from build123d import *

# Parameters (mm, degrees)
SKETCH1_R           = 9
SKETCH1_R_2         = 4
BOSS_EXTRUDE1_DEPTH = 5
SKETCH2_W           = 5
SKETCH2_H           = 10
CUT_EXTRUDE3_DEPTH  = 3
CIRPATTERN1_COUNT   = 6
SKETCH3_R           = 4.05
BOSS_EXTRUDE2_DEPTH = 3


with BuildPart() as part:
    # Sketch1 → Boss-Extrude1 (new body, symmetric)
    with BuildSketch(Plane.XY):
        Circle(SKETCH1_R)
        Circle(SKETCH1_R_2, mode=Mode.SUBTRACT)
    extrude(amount=BOSS_EXTRUDE1_DEPTH, both=True)

    # Sketch2 → Cut-Extrude3 (cut)
    with BuildSketch(Plane(origin=(-9, -17.193061184, 0), x_dir=(0, -1, 0), z_dir=(1, 0, 0))):
        with Locations((-17.193061184, 0)):
            Rectangle(SKETCH2_W, SKETCH2_H)
    cut_extrude3 = extrude(amount=CUT_EXTRUDE3_DEPTH, mode=Mode.SUBTRACT)

    # CirPattern1: Cut-Extrude3 ×6 about axis
    cirpattern1_axis = Axis((0, 0, 0), (0, 0, 1))
    for i in range(1, CIRPATTERN1_COUNT):
        add(cut_extrude3.rotate(cirpattern1_axis, i * 360 / CIRPATTERN1_COUNT), mode=Mode.SUBTRACT)

    # Sketch3 → Boss-Extrude2 (add)
    with BuildSketch(Plane(origin=(-6, 0, 0), x_dir=(0, -1, 0), z_dir=(-1, 0, 0))):
        Circle(SKETCH3_R)
    extrude(amount=BOSS_EXTRUDE2_DEPTH)


solid = part.part
Part model, mm, in its own coordinate system. A direction names the side the tool comes from. Give positions to 0.01 mm unless a question says otherwise; leave off trailing zeros. Order: outer loops, then holes, each group sorted by start corner. A loop starts at its lowest first (then second) coordinate and runs counter-clockwise, first axis right, second up. Notation, with made-up numbers: (50, 46) -> (106, 46) arc R24 ccw to (106, 60) -> close; hole circle Ø1 at (82, 13). An arc over 180 degrees is marked (long way). Use one line per item in the form item = value.
(1) Saw through at D-D (y = -6). Write the cut outline in (x, z), then the cut area to 3 significant figures.
Solution:
outline = (-6.71, -5) -> (-6.35, -5) -> (-6.35, 5) -> (-6.71, 5) -> close; (-1.61, -5) -> (1.61, -5) -> (1.61, 5) -> (-1.61, 5) -> close; (6.35, -5) -> (6.71, -5) -> (6.71, 5) -> (6.35, 5) -> close
area = 39.3 mm²
(2) Saw through at C-C (z = 4.75). Write the cut outline in (x, y), then the cut area to 3 significant figures.
Solution:
outline = (-8.65, -2.5) arc R9 ccw to (-6.49, -6.24) -> (-5.17, -3.95) -> (-0.83, -6.45) -> (-2.16, -8.74) arc R9 ccw to (2.16, -8.74) -> (0.83, -6.45) -> (5.17, -3.95) -> (6.49, -6.24) arc R9 ccw to (8.65, -2.5) -> (6, -2.5) -> (6, 2.5) -> (8.65, 2.5) arc R9 ccw to (6.49, 6.24) -> (5.17, 3.95) -> (0.83, 6.45) -> (2.16, 8.74) arc R9 ccw to (-2.16, 8.74) -> (-0.83, 6.45) -> (-5.17, 3.95) -> (-6.49, 6.24) arc R9 ccw to (-8.65, 2.5) -> (-6, 2.5) -> (-6, -2.5) -> close; hole circle Ø8 at (0, 0)
area = 118 mm²
(3) Tool access for faces 1 (the face through (-5.836, -5.108, 0.07)), 2 (the face through (-7.558, -4.887, 0.07)), 3 (the face through (-6, 0, -4.3)), 4 (the face through (-2.97, 5.214, -0.07)), 5 (the face through (-1.5, -7.6, 0.1)): list every direction of +Z, -Z, +X, -X, +Y, -Y with a clear straight run to the whole face (end or side of a thin tool).
Solution:
face_1 = +Z, -Z, -Y
face_2 = -X, -Y
face_3 = -Z, -X
face_4 = +Z, -Z
face_5 = +Z, -Z, -X
(4) Saw through at A-A (x = 0). Write the cut outline in (y, z), then the cut area to 3 significant figures.
Solution:
outline = (-9, -5) -> (-4, -5) -> (-4, 5) -> (-9, 5) -> close; (4, -5) -> (9, -5) -> (9, 5) -> (4, 5) -> close
area = 100 mm²
(5) Drill centre lines: line 1 (Y direction, x = 0, z = -1); line 2 (X direction, y = 4.5, z = -3); line 3 (X direction, y = -6, z = 2.75). Where is each one in solid material? Low to high. Write a range as from..to.
Solution:
line_1 = -9..-4, 4..9
line_2 = -7.79..-5.48, -4.21..4.21, 5.48..7.79
line_3 = -6.71..-6.35, -1.61..1.61, 6.35..6.71
(6) Saw through at B-B (y = 0). Write the cut outline in (x, z), then the cut area to 3 significant figures.
Solution:
outline = (-9, -4.05) -> (-6, -4.05) -> (-6, -5) -> (-4, -5) -> (-4, 5) -> (-6, 5) -> (-6, 4.05) -> (-9, 4.05) -> close; (4, -5) -> (6, -5) -> (6, 5) -> (4, 5) -> close
area = 64.3 mm²
(7) Flat gauge pins, fed straight in: P1, Ø2.5, axis at y = -0.5, z = 1.5, coming from the +X side; P2, Ø0.5, axis at y = 0, z = 4.5, coming from the -X side; P3, Ø0.9, axis at x = -7.5, z = -4, coming from the +Y side; P4, Ø5, axis at x = 0, y = 0, coming from the +Z side. Where does each tip first touch, or does it go through?
Solution:
P1 = 6
P2 = -6
P3 = 5.59
P4 = through
(8) Pull direction X, two halves, no side cores. Call faces 6 (the face through (7, -2.5, 0)), 7 (the face through (2.97, -5.214, -0.07)), 8 (the face through (5.836, 5.108, 0.07)), 9 (the face through (1.5, -7.6, 0.1)): +X half, -X half, draft (parallel to the pull), parting line (faces both ways), or undercut.
Solution:
face_6 = draft
face_7 = undercut
face_8 = undercut
face_9 = +X half
